Can you work these out from the model? Positions are in its coordinate system, mm. Give positions to 0.01 mm unless a question says otherwise; leave off trailing zeros. Order: outer loops, then holes, each group sorted by start corner. A loop starts at its lowest first (then second) coordinate and runs counter-clockwise, first axis right, second up. Notation, with made-up numbers: (-32.75, 23) - (12.25, 23) arc R8 ccw to (12.25, 31) - close; hole circle Ø3 at (-20, 77.25). An arc over 180 degrees is marked (long way). Answer as a JSON object with one key per item and string values.
```python
from build123d import *

# Parameters (mm, degrees)
SKETCH1_R                        = 1.6383
BOSS_EXTRUDE1_DEPTH              = 1.575
CUT_EXTRUDE1_DEPTH               = 2.54
CUTOUTS_FOR_THRUSTER_HEADS_DEPTH = 1.575
NOTCH_FOR_BPR_TOP_VIEW_W         = 2.575
NOTCH_FOR_BPR_TOP_VIEW_H         = 6.27
CUT_EXTRUDE11_DEPTH              = 10
NOTCH_FOR_BPL_TOP_VIEW_W         = 2.575
NOTCH_FOR_BPL_TOP_VIEW_H         = 6.27
CUT_EXTRUDE12_DEPTH              = 65.400936523
SKETCH22_W                       = 1.501374709
SKETCH22_H                       = 61.468
SKETCH22_W_2                     = 1.585
BOSS_EXTRUDE2_DEPTH              = 1.575
SKETCH23_W                       = 7.1002401
SKETCH23_H                       = 1.27
SKETCH23_W_2                     = 7.016
CUT_EXTRUDE13_DEPTH              = 65.400936523


with BuildPart() as part:
    # Sketch1 → Boss-Extrude1 (new body)
    with BuildSketch(Plane(origin=(0, 0, 0), x_dir=(1, 0, 0), z_dir=(0, 1, 0))):
        with BuildLine():
            Line((-44, 45), (-44, 29.162404323))
            ThreePointArc((-44, 29.162404323), (-43.886381258, 28.888104416), (-43.612081351, 28.774485674))
            Line((-43.612081351, 28.774485674), (-33.211918649, 28.774485674))
            ThreePointArc((-33.211918649, 28.774485674), (-32.937618742, 28.660866933), (-32.824, 28.386567026))
            Line((-32.824, 28.386567026), (-32.824, -32.305595677))
            ThreePointArc((-32.824, -32.305595677), (-32.937618742, -32.579895584), (-33.211918649, -32.693514326))
            Line((-33.211918649, -32.693514326), (-36.100000052, -32.693514326))
            Line((-36.100000052, -32.693514326), (-43.612081299, -32.693514326))
            ThreePointArc((-43.612081299, -32.693514326), (-43.886381206, -32.807133067), (-43.999999948, -33.081432974))
            Line((-43.999999948, -33.081432974), (-43.999999948, -38.977))
            Line((-43.999999948, -38.977), (-43.999999948, -45))
            ThreePointArc((-43.999999948, -45), (-43.41421351, -46.414213562), (-41.999999948, -47))
            Line((-41.999999948, -47), (42.705916546, -47))
            Line((42.705916546, -47), (43.849731117, -47))
            Line((43.849731117, -47), (43.849731117, -38.27))
            Line((43.849731117, -38.27), (43.849731117, -33.081432974))
            ThreePointArc((43.849731117, -33.081432974), (43.736112376, -32.807133067), (43.461812469, -32.693514326))
            Line((43.461812469, -32.693514326), (36.098785193, -32.693514326))
            Line((36.098785193, -32.693514326), (33.824, -32.693514326))
            Line((33.824, -32.693514326), (32.822785141, -32.693514326))
            Line((32.822785141, -32.693514326), (32.822785141, -30.469351623))
            Line((32.822785141, -30.469351623), (32.822785141, 27.774485674))
            ThreePointArc((32.822785141, 27.774485674), (33.11567836, 28.481592456), (33.822785141, 28.774485674))
            Line((33.822785141, 28.774485674), (43.611054239, 28.774485674))
            ThreePointArc((43.611054239, 28.774485674), (43.885287743, 28.88803803), (43.998972842, 29.162216531))
            Line((43.998972842, 29.162216531), (44, 31.284))
            Line((44, 31.284), (44, 45))
            ThreePointArc((44, 45), (43.414213562, 46.414213562), (42, 47))
            Line((42, 47), (-42, 47))
            ThreePointArc((-42, 47), (-43.414213562, 46.414213562), (-44, 45))
        make_face()
        with Locations(Location((40, 43.5, 0), (0, 0, 270))):
            Circle(SKETCH1_R, mode=Mode.SUBTRACT)
        with Locations(Location((-40, 43.5, 0), (0, 0, 270))):
            Circle(SKETCH1_R, mode=Mode.SUBTRACT)
        with Locations(Location((-37.599999948, -42.2, 0), (0, 0, 270))):
            Circle(SKETCH1_R, mode=Mode.SUBTRACT)
        with Locations(Location((36.100000052, -42.2, 0), (0, 0, 270))):
            Circle(SKETCH1_R, mode=Mode.SUBTRACT)
        Polygon((23.409, -31.5), (-23.409, -31.5), (-23.409, 13.29544), (-12.909, 13.29544), (-12.909, 25.99544), (12.909, 25.99544), (12.909, 13.29544), (23.409, 13.29544), align=None, mode=Mode.SUBTRACT)
    extrude(amount=BOSS_EXTRUDE1_DEPTH)

    # Sketch2 → Cut-Extrude1 (cut)
    with BuildSketch(Plane(origin=(0, 1.575, 0), x_dir=(1, 0, 0), z_dir=(0, 1, 0))):
        Polygon((-12.909, 19.06), (-30.435, 19.06), (-30.435, 47), (30.435, 47), (30.435, 19.06), (12.909, 19.06), (12.909, 25.99544), (-12.909, 25.99544), align=None)
    extrude(amount=-CUT_EXTRUDE1_DEPTH, mode=Mode.SUBTRACT)

    # Sketch16 → Cutouts for Thruster Heads (add)
    with BuildSketch(Plane(origin=(0, 1.575, 0), x_dir=(1, 0, 0), z_dir=(0, 1, 0))):
        Polygon((12.909, 19.06), (12.909, 13.29544), (-12.909, 13.29544), (-12.909, 19.06), (-30.435, 19.06), (-30.435, 21), (-11.838888217, 21), (-11.838888217, 47), (11.909, 47), (11.909, 21), (30.435, 21), (30.435, 19.06), align=None)
    extrude(amount=-CUTOUTS_FOR_THRUSTER_HEADS_DEPTH)

    # Notch for BPR (TOP VIEW) → Cut-Extrude11 (cut)
    with BuildSketch(Plane(origin=(0, 1.575, 0), x_dir=(1, 0, 0), z_dir=(0, 1, 0))):
        with Locations((-35.6965, 31.909485674)):
            Rectangle(NOTCH_FOR_BPR_TOP_VIEW_W, NOTCH_FOR_BPR_TOP_VIEW_H)
    extrude(amount=-CUT_EXTRUDE11_DEPTH, mode=Mode.SUBTRACT)

    # Notch for BPL (TOP VIEW) → Cut-Extrude12 (cut, through all)
    with BuildSketch(Plane(origin=(0, 1.575, 0), x_dir=(1, 0, 0), z_dir=(0, 1, 0))):
        with Locations((35.61165985, 31.909485674)):
            Rectangle(NOTCH_FOR_BPL_TOP_VIEW_W, NOTCH_FOR_BPL_TOP_VIEW_H)
    extrude(amount=-CUT_EXTRUDE12_DEPTH, mode=Mode.SUBTRACT)

    # Sketch22 → Boss-Extrude2 (add)
    with BuildSketch(Plane(origin=(0, 1.575, 0), x_dir=(1, 0, 0), z_dir=(0, 1, 0))):
        with Locations((33.573472495, -1.959514326)):
            Rectangle(SKETCH22_W, SKETCH22_H)
        with Locations((-33.6165, -1.959514326)):
            Rectangle(SKETCH22_W_2, SKETCH22_H)
    extrude(amount=-BOSS_EXTRUDE2_DEPTH)

    # Sketch23 → Cut-Extrude13 (cut, through all)
    with BuildSketch(Plane(origin=(0, 1.575, 0), x_dir=(1, 0, 0), z_dir=(0, 1, 0))):
        with Locations((40.4492799, 29.409485674)):
            Rectangle(SKETCH23_W, SKETCH23_H)
        with Locations((-40.492, 29.409485674)):
            Rectangle(SKETCH23_W_2, SKETCH23_H)
    extrude(amount=-CUT_EXTRUDE13_DEPTH, mode=Mode.SUBTRACT)


solid = part.part
```
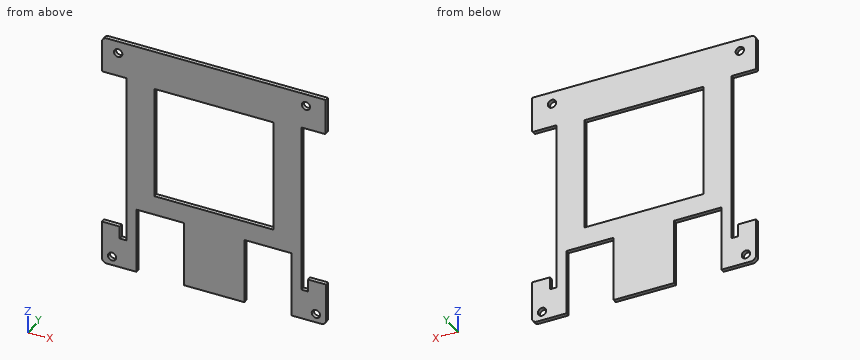
Q1. If we section it at A-A, the plane x = -7.5: Please give me the cut outline in (y, z) (3 decimals), then the cut area to 3 significant figures.
Recorded:
{"outline": "(0, -47) - (1.575, -47) - (1.575, -13.295) - (0, -13.295) - close; (0, 31.5) - (1.575, 31.5) - (1.575, 47) - (0, 47) - close", "area": "77.5 mm^2"}
Q2. I'm going to push flat-ended pins straight in: pin 1 Ø3 at (x, z) = (-37.6, 42.2) entering from -Y; pin 2 Ø0.5 at (y, z) = (1, -29.5) entering from +X; pin 3 Ø0.8 at (x, y) = (22, 0.5) entering from -Z. Where does each tip first touch, or does it pass through?
Recorded:
{"pin 1": "passes through", "pin 2": "stops at x = 34.32", "pin 3": "stops at z = -21"}
Q3. If we section it at D-D, the plane x = 40: Please give me the cut outline in (y, z) (3 decimals), then the cut area to 3 significant figures.
Recorded:
{"outline": "(0, -47) - (1.575, -47) - (1.575, -45.138) - (0, -45.138) - close; (0, -41.862) - (1.575, -41.862) - (1.575, -30.044) - (0, -30.044) - close; (0, 32.694) - (1.575, 32.694) - (1.575, 47) - (0, 47) - close", "area": "44.1 mm^2"}
Q4. If we section it at B-B, the plane z = 3: Please give me the cut outline in (x, y) (3 decimals).
Recorded:
{"outline": "(-34.409, 0) - (-23.409, 0) - (-23.409, 1.575) - (-34.409, 1.575) - close; (23.409, 0) - (34.324, 0) - (34.324, 1.575) - (23.409, 1.575) - close"}
Q5. If we section it at C-C, the plane z = 42.2: Please give me the cut outline in (x, y) (3 decimals).
Recorded:
{"outline": "(-44, 0) - (-39.238, 0) - (-39.238, 1.575) - (-44, 1.575) - close; (-35.962, 0) - (34.462, 0) - (34.462, 1.575) - (-35.962, 1.575) - close; (37.738, 0) - (43.85, 0) - (43.85, 1.575) - (37.738, 1.575) - close"}
Q6. I need wall thicknesses on L1, parallel to X at y = 0.4, z = -40.5 (3 decimals); L2, parallel to X at y = 1.25, z = 42.2; L3, parallel to X at y = 1.1, z = -43.5 (3 decimals). Which ranges of each line are inside material? Lowest first, please.
Recorded:
{"L1": "x = -44 to -30.435, -11.839 to 11.909, 30.435 to 44", "L2": "x = -44 to -39.24, -35.96 to 34.46, 37.74 to 43.85", "L3": "x = -44 to -41.638, -38.362 to -30.435, -11.839 to 11.909, 30.435 to 38.362, 41.638 to 44"}
